Part print with two shaded views. Sizes in mm from the minimum x, y, z corner. A direction names the side the tool comes from. Round coordinates to 2 decimals unless told otherwise and drop trailing zeros. Order: outer loops, then holes, each group sorted by start corner. A loop starts at its lowest first (then second) coordinate and runs counter-clockwise, first axis right, second up. Notation, with made-up numbers: (74, -19.75) - (124, -19.75) arc R22 ccw to (124, 19.25) - close; hole circle Ø10 at (77.25, -38). An arc over 180 degrees is marked (long way). Answer as CSV lines item,"result". Start each with the question number.
1. Band-saw the part on A-A on z = 30.5. List the corners of the cut face in (x, y), then the cut area to 3 significant figures.
2. 3-axis set-ups, long thin cutter, end or side, ignore diameter. For the marked faces 1 and 2: which of +Z, -Z, +X, -X, +Y, -Y reach the whole face in a straight line?
3. Wall check: line 1 along Y through (x, z) = (9, 1.05); line 2 along Y through (x, z) = (56, 1.2); line 3 along Z through (x, y) = (57, 23). Give the ranges that are in metal, low to high. Write a range as [from, to].
4. Band-saw the part on B-B on y = 15.5. List the corners of the cut face in (x, z), then the cut area to 3 significant figures.
5. Band-saw the part on C-C on x = 32.5. List the corners of the cut face in (y, z).
6. Pin check, flat tips, straight feed: pin 1 Ø5 at (x, z) = (40, 10) entering from +Y; pin 2 Ø4 at (x, y) = (9, 15.5) entering from +Z; pin 3 Ø7 at (x, y) = (56, 15.5) entering from +Z. Stop position of each tip, or through.
7. Band-saw the part on D-D on y = 39. List the corners of the cut face in (x, z), then the cut area to 3 significant figures.
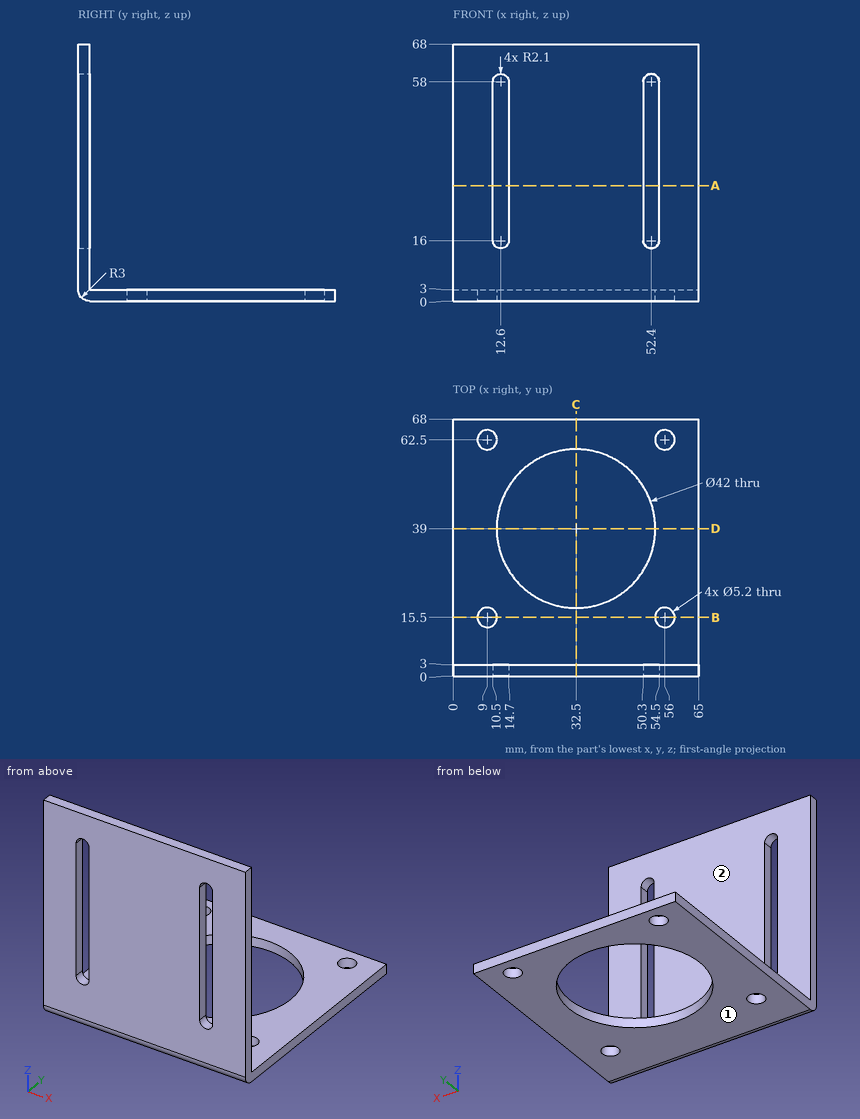
Reply:
1,outline,"(0, 0) - (10.5, 0) - (10.5, 3) - (0, 3) - close; (14.7, 0) - (50.3, 0) - (50.3, 3) - (14.7, 3) - close; (54.5, 0) - (65, 0) - (65, 3) - (54.5, 3) - close"
1,area,"170 mm2"
2,face 1,"-Z, +X, -X, +Y, -Y"
2,face 2,"+Z, +X, -X, +Y"
3,line 1,"y = [0.72, 12.9], [18.1, 59.9], [65.1, 68]"
3,line 2,"y = [0.6, 12.9], [18.1, 59.9], [65.1, 68]"
3,line 3,"z = [0, 3]"
4,outline,"(0, 0) - (6.4, 0) - (6.4, 3) - (0, 3) - close; (11.6, 0) - (53.4, 0) - (53.4, 3) - (11.6, 3) - close; (58.6, 0) - (65, 0) - (65, 3) - (58.6, 3) - close"
4,area,"164 mm2"
5,outline,"(0, 3) arc R3 ccw to (3, 0) - (18, 0) - (18, 3) - (3, 3) - (3, 68) - (0, 68) - close; (60, 0) - (68, 0) - (68, 3) - (60, 3) - close"
6,pin 1,"stops at y = 3"
6,pin 2,"passes through"
6,pin 3,"stops at z = 3"
7,outline,"(0, 0) - (11.5, 0) - (11.5, 3) - (0, 3) - close; (53.5, 0) - (65, 0) - (65, 3) - (53.5, 3) - close"
7,area,"69.0 mm2"
